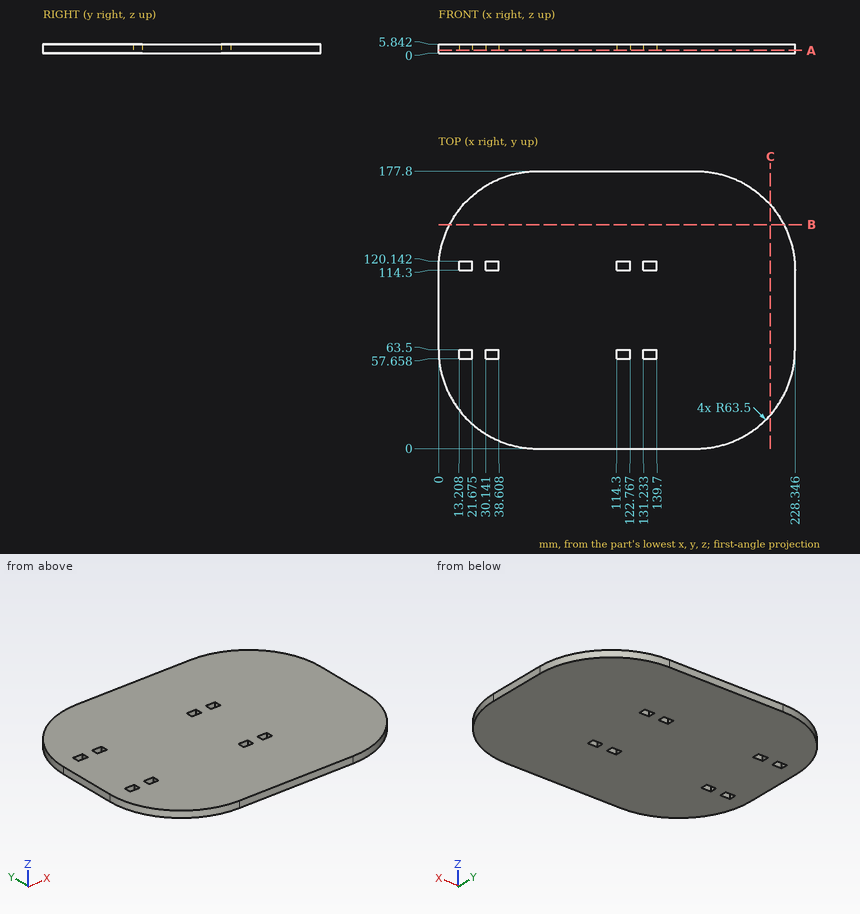
Source: three-view drawing plus pictorial views. Frame: mm from the lowest corner of the part. Round coordinates to 2 decimals unless told otherwise and drop trailing zeros. Write each loop counter-clockwise with the first axis right and the second up, starting at its lowest first coordinate (ties: lowest second). Pieces come first, ordered by that corner, then holes. Notation, with made-up numbers: M 18.5,6.5 L 33.5,6.5 A15 cw 33.5,28.5 Z; hole C 89.5,79 d11. An arc over 180 degrees is marked long. Write each question's results on one line, items separated by ' | '.
Q1. Line query: line 1 along X through (y, z) = (62.5, 1.65) (1 decimal); line 2 along Y through (x, z) = (117.5, 0.55); line 3 along X through (y, z) = (117.5, 4.6) (1 decimal). Output: solid intervals per line, ascending.
Results:
line 1: x = 0 to 13.2, 21.7 to 30.1, 38.6 to 114.3, 122.8 to 131.2, 139.7 to 228.3 | line 2: y = 0 to 57.66, 63.5 to 114.3, 120.14 to 177.8 | line 3: x = 0.1 to 13.2, 21.7 to 30.1, 38.6 to 114.3, 122.8 to 131.2, 139.7 to 228.3
Q2. Pin query (flat end, axial travel): P1, Ø1.8, axis at y = 60, z = 4, coming from the -X side; P2, Ø1.8, axis at y = 59.5, z = 2.5, coming from the +X side; P3, Ø3, axis at x = 15.5, z = 3, coming from the +Y side. Return the tip coordinate at first contact, or that it passes through.
Results:
P1: stops at x = 0.05 | P2: stops at x = 228.27 | P3: stops at y = 157.54
Q3. Section query C-C (x = 212.5). Return loops of the section in (y, z).
Results:
outline: M 21.53,0 L 156.27,0 L 156.27,5.84 L 21.53,5.84 Z
Q4. Section query A-A (z = 1.8). State how many separate pieces and enclosed holes the cut face has, and give its area (3 significant figures).
Results:
separate pieces: 1 | enclosed holes: 8 | area: 36,700 mm^2
Q5. Section query B-B (y = 143.5). Return loops of the section in (x, z), and give its area (3 significant figures).
Results:
outline: M 7.11,0 L 221.23,0 L 221.23,5.84 L 7.11,5.84 Z | area: 1,250 mm^2
